```python
from build123d import *

# Parameters (mm, degrees)
SKETCH_1_W         = 8
SKETCH_1_H         = 8
EXTRUDE_1_DEPTH    = 24
HOLE_WIZARD_M3_1_D = 2.5
HOLE_WIZARD_M3_2_D = 2.5
HOLE_WIZARD_M3_3_D = 2.5


with BuildPart() as part:
    # 草图1 → 凸台-拉伸1 (new, symmetric)
    with BuildSketch(Plane(origin=(0, 0, 0), x_dir=(1, 0, 0), z_dir=(0, 1, 0))):
        Rectangle(SKETCH_1_W, SKETCH_1_H)
    extrude(amount=EXTRUDE_1_DEPTH, both=True)

    # M3 螺纹孔1 (through all)
    with Locations(Plane.XY.offset(4)):
        with Locations((0, 8), (0, -8)):
            Hole(HOLE_WIZARD_M3_1_D / 2)

    # M3 螺纹孔2 (through all)
    with Locations(Plane(origin=(4, 0, 0), x_dir=(0, 0, -1), z_dir=(1, 0, 0))):
        with Locations((0, 16), (0, -16)):
            Hole(HOLE_WIZARD_M3_2_D / 2)

    # M3 螺纹孔3 (through all)
    with Locations(Plane(origin=(0, -24, 0), x_dir=(-1, 0, 0), z_dir=(0, -1, 0))):
        with Locations((0, 0)):
            Hole(HOLE_WIZARD_M3_3_D / 2)


solid = part.part
```
Read the model definition and answer for the solid it produces. Units are mm, in the model's axes. Round coordinates to 2 decimals unless told otherwise and drop trailing zeros. Write each loop counter-clockwise with the first axis right and the second up, starting at its lowest first coordinate (ties: lowest second). Pieces come first, ordered by that corner, then holes. Notation, with made-up numbers: (19.5, -12.75) - (78.5, -12.75) arc R23 cw to (78.5, 7.25) - close; hole circle Ø1 at (-35.75, 8). An arc over 180 degrees is marked (long way). Use CSV: the item, a comma, the result in double quotes.
Q1. Straight lines are drawn through the part: line 1 along Y through (x, z) = (0, -3.1); line 2 along Y through (x, z) = (2.7, 0); line 3 along X through (y, z) = (8, -2.3). For each, find the intervals that lie inside material, in ascending order.
Values:
line 1,"y = -24 to -9.25, -6.75 to 6.75, 9.25 to 24"
line 2,"y = -24 to -17.25, -14.75 to 14.75, 17.25 to 24"
line 3,"x = -4 to -1.25, 1.25 to 4"
Q2. Find section D-D, the plane z = -0.5. Count the separate pieces of the cut face and the enclosed holes in it, then the cut area to 3 significant figures.
Values:
separate pieces,"6"
enclosed holes,"0"
area,"248 mm²"
Q3. Find section C-C, the plane y = -11. Write down the section's boundary in (x, z), then the cut area to 3 significant figures.
Values:
outline,"(-4, -4) - (4, -4) - (4, 4) - (-4, 4) - close; hole circle Ø2.5 at (0, 0)"
area,"59.1 mm²"
Q4. Each of these flat-tipped pins is pushed along its axis until it touches: pin 1 Ø4 at (y, z) = (-16, 0) entering from -X; pin 2 Ø2 at (x, y) = (0, 8) entering from -Z. Where does it stop, or does it pass through?
Values:
pin 1,"stops at x = -4"
pin 2,"passes through"
Q5. Determine the mould class of faces 1 (the cylindrical face through (-1.25, -19.94, -0.05)), 2 (the flat face through (4, 0, 0)), 3 (the flat face through (0, 0, -4)) for opening direction X: +X half, -X half, draft (parallel to the pull), parting line (faces both ways), or undercut.
Values:
face 1,"undercut"
face 2,"+X half"
face 3,"draft"
Q6. Find section B-B, the plane x = 3.25. Write down the section's boundary in (y, z).
Values:
outline,"(-24, -4) - (24, -4) - (24, 4) - (-24, 4) - close; hole circle Ø2.5 at (-16, 0); hole circle Ø2.5 at (16, 0)"
Q7. Find section A-A, the plane z = 1.75. Write down the section's boundary in (x, y).
Values:
outline,"(-4, -24) - (4, -24) - (4, 24) - (-4, 24) - close; hole circle Ø2.5 at (0, -8); hole circle Ø2.5 at (0, 8)"
